Verification items for the finished model (mm, model axes). Round coordinates to 2 decimals unless told otherwise and drop trailing zeros. One line per item, written item: value.
from build123d import *

# Parameters (mm, degrees)
F0_R     = 2.5
F1_DEPTH = 1.25
F2_R     = 2.49999
F3_SIZE  = 1.5


# Not quite as in the source:
# - a fillet or chamfer is up to 0.001 mm smaller than in the source, because OpenCascade refuses the exact size


with BuildPart() as f1:
    # F0 (on Top) → F1 (new body, symmetric)
    with BuildSketch(Plane.XY):
        Polygon((41.4534954924, 86.8201051839), (-41.4535404544, 86.8201051839), (-41.4535404544, -23.9118914119), (21.4531252731, -86.8199001066), (41.4534954924, -86.8199001066), align=None)
        with BuildLine():
            ThreePointArc((-25.0127278268, -26.2106563896), (-21.4771550521, -24.7462917212), (-17.9416265813, -26.210763353))
            Line((-17.9416265813, -26.210763353), (14.5847404845, -58.7378248101))
            ThreePointArc((14.5847404845, -58.7378248101), (16.0492105587, -62.2733815916), (14.5847972009, -65.8089618652))
            Line((14.5847972009, -65.8089618652), (12.816990028, -67.5766218932))
            ThreePointArc((12.816990028, -67.5766218932), (9.2814327639, -69.0409837172), (5.745914741, -67.5765271526))
            Line((5.745914741, -67.5765271526), (-26.7805685052, -35.0493495125))
            ThreePointArc((-26.7805685052, -35.0493495125), (-28.2451162288, -31.5138612573), (-26.7805848271, -27.9783662409))
            Line((-26.7805848271, -27.9783662409), (-25.0127278268, -26.2106563896))
        make_face(mode=Mode.SUBTRACT)
        with Locations((-36.4535404544, -8.1798948161)):
            Circle(F0_R, mode=Mode.SUBTRACT)
        with Locations((36.4534954924, -71.8298948161)):
            Circle(F0_R, mode=Mode.SUBTRACT)
        with Locations((36.4534954924, -1.2798948161)):
            Circle(F0_R, mode=Mode.SUBTRACT)
        with BuildLine():
            Line((-20.7271233506, -3.1984749304), (-20.7271233506, 69.3290029653))
            ThreePointArc((-20.7271233506, 69.3290029653), (-17.1909981799, 67.8582257506), (-15.7271233506, 64.3192375729))
            Line((-15.7271233506, 64.3192375729), (-15.7271233506, -8.1786223686))
            ThreePointArc((-15.7271233506, -8.1786223686), (-19.2614484064, -6.7269968768), (-20.7271233506, -3.1984749304))
        make_face(mode=Mode.SUBTRACT)
        with BuildLine():
            Line((-2.5021233506, -3.1984749304), (-2.5021233506, 69.3290029653))
            ThreePointArc((-2.5021233506, 69.3290029653), (1.0340018201, 67.8582257506), (2.4978766494, 64.3192375729))
            Line((2.4978766494, 64.3192375729), (2.4978766494, -8.1786223686))
            ThreePointArc((2.4978766494, -8.1786223686), (-1.0364484064, -6.7269968768), (-2.5021233506, -3.1984749304))
        make_face(mode=Mode.SUBTRACT)
        with Locations((-36.4535404544, 69.3201051839)):
            Circle(F0_R, mode=Mode.SUBTRACT)
        with BuildLine():
            Line((15.7228766494, -3.1984749304), (15.7228766494, 69.3290029653))
            ThreePointArc((15.7228766494, 69.3290029653), (19.2590018201, 67.8582257506), (20.7228766494, 64.3192375729))
            Line((20.7228766494, 64.3192375729), (20.7228766494, -8.1786223686))
            ThreePointArc((20.7228766494, -8.1786223686), (17.1885515936, -6.7269968768), (15.7228766494, -3.1984749304))
        make_face(mode=Mode.SUBTRACT)
        with Locations((36.4534954924, 69.3201051839)):
            Circle(F0_R, mode=Mode.SUBTRACT)
    extrude(amount=F1_DEPTH, both=True)

    # F2 (radius 2.5 in the source; OpenCascade refuses exactly that, so slightly less here)
    f2_edges = [f1.edges().sort_by_distance(p)[0] for p in [
        (-10.517327, -51.312938, 1.25),
        (-20.727123, 33.065264, 1.25),
        (-2.502123, 33.065264, 1.25),
        (15.722877, 33.065264, 1.25),
        (-17.190998, 67.858226, 1.25),
        (1.034002, 67.858226, 1.25),
        (19.259002, 67.858226, 1.25),
        (-2.2e-05, 86.820105, 1.25),
    ]]
    fillet(f2_edges, radius=F2_R)

    # F3
    f3_edges = [f1.edges().sort_by_distance(p)[0] for p in [
        (-38.95354, -8.179895, 1.25),
        (-38.95354, 69.320105, 1.25),
        (33.953495, 69.320105, 1.25),
        (33.953495, -1.279895, 1.25),
        (33.953495, -71.829895, 1.25),
    ]]
    chamfer(f3_edges, length=F3_SIZE)


solid = f1.part
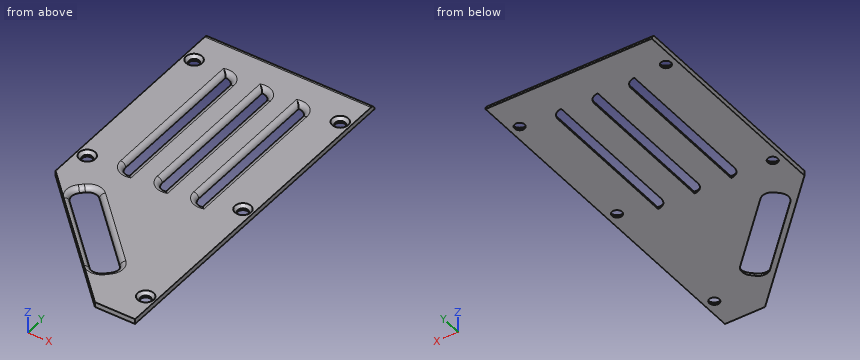
(1) Thickness scan on L1, parallel to X at y = 18, z = -1.05; L2, parallel to X at y = -8.5, z = -0.95; L3, parallel to X at y = -6, z = 0.1. Record the ranges inside material, lowest first. Write a range as from..to.
Completed:
L1: x = -41.45..-20.74, -15.72..-2.51, 2.51..15.71, 20.73..41.45
L2: x = -41.45..-38.93, -33.97..41.45
L3: x = -41.45..-38.29, -34.62..-20.34, -15.33..-2.11, 2.89..16.11, 21.12..41.45
(2) Sectioned sample at A-A on y = 19. Count the separate pieces of the cut face and the enclosed holes in it, and give its area (3 significant figures).
Completed:
separate pieces: 4
enclosed holes: 0
area: 162 mm^2
(3) Depth check by flat-ended pin: pin 1 Ø4 at (x, y) = (-16.5, 1.5) entering from +Z; pin 2 Ø6 at (x, y) = (-36.45, -8.18) entering from +Z; pin 3 Ø1.5 at (x, z) = (-7.5, 0) entering from -Y. Enter the tip coordinate at first touch or a pass-through.
Completed:
pin 1: stops at z = 0.9
pin 2: stops at z = 0.25
pin 3: stops at y = -58.62
